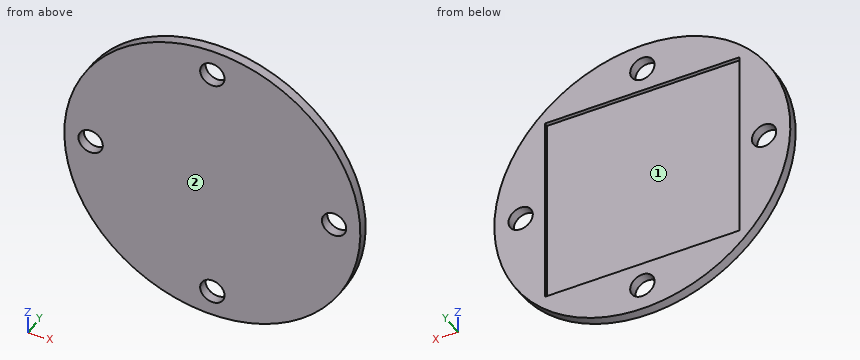
from build123d import *

# Parameters (mm, degrees)
SKETCH1_R           = 76
SKETCH1_W           = 100
SKETCH1_H           = 100
BOSS_EXTRUDE1_DEPTH = 5
SKETCH3_W           = 100
SKETCH3_H           = 100
BOSS_EXTRUDE2_DEPTH = 5
SKETCH3_2_W         = 100
SKETCH3_2_H         = 100
CUT_EXTRUDE1_DEPTH  = 2
SKETCH6_R           = 6.25
CUT_EXTRUDE2_DEPTH  = 10


with BuildPart() as part:
    # Sketch1 → Boss-Extrude1 (new body)
    with BuildSketch(Plane(origin=(0, 0, 0), x_dir=(1, 0, 0), z_dir=(0, 1, 0))):
        with Locations(Location((0, 0, 0), (0, 0, 270))):
            Circle(SKETCH1_R)
        Rectangle(SKETCH1_W, SKETCH1_H, mode=Mode.SUBTRACT)
    extrude(amount=BOSS_EXTRUDE1_DEPTH)

    # Sketch3 → Boss-Extrude2 (add)
    with BuildSketch(Plane(origin=(0, 5, 0), x_dir=(1, 0, 0), z_dir=(0, 1, 0))):
        Rectangle(SKETCH3_W, SKETCH3_H)
    extrude(amount=-BOSS_EXTRUDE2_DEPTH)

    # Sketch3_2 → Cut-Extrude1 (cut)
    with BuildSketch(Plane(origin=(0, 5, 0), x_dir=(1, 0, 0), z_dir=(0, 1, 0))):
        Rectangle(SKETCH3_2_W, SKETCH3_2_H)
    extrude(amount=-CUT_EXTRUDE1_DEPTH, mode=Mode.SUBTRACT)

    # Sketch6 → Cut-Extrude2 (cut)
    with BuildSketch(Plane(origin=(0, 5, 0), x_dir=(1, 0, 0), z_dir=(0, 1, 0))):
        with Locations(Location((0, 62.5, 0), (0, 0, 270))):
            Circle(SKETCH6_R)
        with Locations(Location((62.5, 0, 0), (0, 0, 270))):
            Circle(SKETCH6_R)
        with Locations(Location((0, -62.5, 0), (0, 0, 270))):
            Circle(SKETCH6_R)
        with Locations(Location((-62.5, 0, 0), (0, 0, 270))):
            Circle(SKETCH6_R)
    extrude(amount=-CUT_EXTRUDE2_DEPTH, mode=Mode.SUBTRACT)


solid = part.part
Build history of the part. All positions in model axes, mm. Face numbers are marked on the shaded views. A direction names the side the tool comes from. Round coordinates to 2 decimals unless told otherwise and drop trailing zeros. Write each loop counter-clockwise with the first axis right and the second up, starting at its lowest first coordinate (ties: lowest second). Pieces come first, ordered by that corner, then holes. Notation, with made-up numbers: (6, 60.25) -> (38, 60.25) arc R17 ccw to (38, 92.25) -> close; hole circle Ø11 at (-36, 55.25). An arc over 180 degrees is marked (long way). Use one line per item in the form item = value.
Q1. Band-saw the part on B-B, the plane x = 62.5. Write the cut outline in (y, z).
Conclusion:
outline = (0, -43.24) -> (5, -43.24) -> (5, -6.25) -> (0, -6.25) -> close; (0, 6.25) -> (5, 6.25) -> (5, 43.24) -> (0, 43.24) -> close
Q2. Drill centre lines: L1, parallel to X at y = 2.8, z = 0; L2, parallel to X at y = 3.6, z = 1; L3, parallel to X at y = 4.75, z = 5.5. Where is each one in solid material? Low to high.
Conclusion:
L1 = -76 to -68.75, -56.25 to 56.25, 68.75 to 76
L2 = -75.99 to -68.67, -56.33 to -50, 50 to 56.33, 68.67 to 75.99
L3 = -75.8 to -65.47, -59.53 to -50, 50 to 59.53, 65.47 to 75.8
Q3. Drop flat-ended pins along their axis: P1, Ø12, axis at x = 27.5, z = -21.5, coming from the +Y side; P2, Ø0.6, axis at y = 4, z = -20, coming from the -X side; P3, Ø1, axis at x = 22.5, y = 4, coming from the +Z side. Give the stop position or say it passes through.
Conclusion:
P1 = 3
P2 = -73.4
P3 = 72.75
Q4. Band-saw the part on A-A, the plane z = 0. Write the cut outline in (x, y), then the cut area to 3 significant figures.
Conclusion:
outline = (-76, 0) -> (-68.75, 0) -> (-68.75, 5) -> (-76, 5) -> close; (-56.25, 0) -> (56.25, 0) -> (56.25, 5) -> (50, 5) -> (50, 3) -> (-50, 3) -> (-50, 5) -> (-56.25, 5) -> close; (68.75, 0) -> (76, 0) -> (76, 5) -> (68.75, 5) -> close
area = 435 mm²
Q5. Band-saw the part on D-D, the plane y = 1.8. Write the cut outline in (x, z), then the cut area to 3 significant figures.
Conclusion:
outline = circle Ø152 at (0, 0); hole circle Ø12.5 at (-62.5, 0); hole circle Ø12.5 at (0, -62.5); hole circle Ø12.5 at (0, 62.5); hole circle Ø12.5 at (62.5, 0)
area = 17,700 mm²
Q6. Band-saw the part on C-C, the plane z = -62.5. Write the cut outline in (x, y), then the cut area to 3 significant figures.
Conclusion:
outline = (-43.24, 0) -> (-6.25, 0) -> (-6.25, 5) -> (-43.24, 5) -> close; (6.25, 0) -> (43.24, 0) -> (43.24, 5) -> (6.25, 5) -> close
area = 370 mm²
Q7. Tool access for the marked faces 1 and 2: list every direction of +Z, -Z, +X, -X, +Y, -Y with a clear straight run to the whole face (end or side of a thin tool).
Conclusion:
face_1 = +Y
face_2 = +Z, -Z, +X, -X, -Y
